```python
from build123d import *

# Parameters (mm, degrees)
ORIGINAL_TRUSS_PART_DEPTH = 30
SKETCH14_W                = 30
SKETCH14_H                = 30
CENTER_SUPPORT_DEPTH      = 305.758522
RIGHT_SUPPORT_REACH       = 302
SKETCH15_W                = 80
SKETCH15_H                = 30


with BuildPart() as part:
    # Sketch2 → Original Truss Part (new body)
    with BuildSketch(Plane.XY):
        Polygon((0, 0), (-928.915298157, 0), (-928.915298157, 27.120739154), (71.084701843, 27.120739154), (71.084701843, -32.879260846), (-8.915298157, -32.879260846), (-928.915298157, -330), (-928.915298157, -300), align=None)
    original_truss_part = extrude(amount=-ORIGINAL_TRUSS_PART_DEPTH)

    # OG Part Mirror: Original Truss Part across plane
    add(original_truss_part.mirror(Plane.ZX.offset(-152.879260846)))

    # Sketch14 → Center Support (add)
    with BuildSketch(Plane(origin=(0, -305.758521692, 0), x_dir=(1, 0, 0), z_dir=(0, 1, 0))):
        with Locations((-426.927182328, 15)):
            Rectangle(SKETCH14_W, SKETCH14_H)
    extrude(amount=CENTER_SUPPORT_DEPTH)

    # Right Support: up to this plane
    right_support_end = Plane(origin=(-8.915298157, -32.879260846, -30), z_dir=(0.307327428, -0.951603831, 0))
    # Sketch15 → Right Support (add, up to the surface)
    with BuildSketch(Plane(origin=(0, -272.879260846, 0), x_dir=(1, 0, 0), z_dir=(0, 1, 0)), mode=Mode.PRIVATE) as right_support_sk1:
        with Locations((31.084701843, 15)):
            Rectangle(SKETCH15_W, SKETCH15_H)
    right_support_tool1 = split(extrude(right_support_sk1.sketch, amount=RIGHT_SUPPORT_REACH, mode=Mode.PRIVATE), bisect_by=right_support_end, keep=Keep.BOTH, mode=Mode.PRIVATE)
    add(right_support_tool1.solids().sort_by_distance((31.084702, -272.879261, -15))[0])


solid = part.part
```
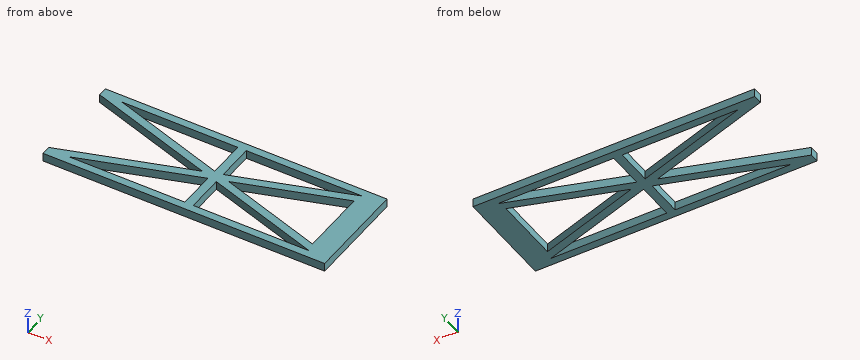
CAD build for the part. Positions are in the model's coordinates, mm. Give positions to 0.01 mm unless a question says otherwise; leave off trailing zeros. Order: outer loops, then holes, each group sorted by start corner. A loop starts at its lowest first (then second) coordinate and runs counter-clockwise, first axis right, second up.
(1) Saw through at C-C, the plane x = -559.5. Give the cut face in (y, z).
(2) Saw through at B-B, the plane y = -189. Give the cut face in (x, z), then the cut area to 3 significant figures.
(3) Saw through at A-A, the plane z = -10. Give the cut face in (x, y), then the cut area to 3 significant figures.
(4) Flat gauge pin, fed straight in: pin 1 (1 mm diameter, centred on x = -161, y = -58, fed in from +Z). Where does the tip first touch, or does it go through?
(5) Drill centre lines: L1, parallel to Y at x = -661, z = -7; L2, parallel to Y at x = -631, z = -17; L3, parallel to Y at x = -388, z = -9.75. Where is each one in solid material? Low to high.
Results found:
1. outline: (-332.88, -30) - (-305.76, -30) - (-305.76, 0) - (-332.88, 0) - close; (-210.69, -30) - (-180.69, -30) - (-180.69, 0) - (-210.69, 0) - close; (-125.06, -30) - (-95.06, -30) - (-95.06, 0) - (-125.06, 0) - close; (0, -30) - (27.12, -30) - (27.12, 0) - (0, 0) - close
2. outline: (-585.22, -30) - (-492.33, -30) - (-492.33, 0) - (-585.22, 0) - close; (-441.93, -30) - (-411.93, -30) - (-411.93, 0) - (-441.93, 0) - close; (-361.53, -30) - (-268.64, -30) - (-268.64, 0) - (-361.53, 0) - close; (-8.92, -30) - (71.08, -30) - (71.08, 0) - (-8.92, 0) - close
2. area: 8,870 mm2
3. outline: (-928.92, -332.88) - (71.08, -332.88) - (71.08, 27.12) - (-928.92, 27.12) - (-928.92, -5.76) - (-473.37, -152.88) - (-928.92, -300) - close; hole (-853.85, -305.76) - (-441.93, -305.76) - (-441.93, -172.72) - close; hole (-853.85, 0) - (-441.93, -133.03) - (-441.93, 0) - close; hole (-411.93, -305.76) - (0, -305.76) - (-411.93, -172.72) - close; hole (-411.93, -133.03) - (0, 0) - (-411.93, 0) - close; hole (-380.48, -152.88) - (-8.92, -272.88) - (-8.92, -32.88) - close
3. area: 139,000 mm2
4. pin 1: stops at z = 0
5. L1: y = -332.88 to -305.76, -243.47 to -213.47, -92.28 to -62.28, 0 to 27.12
5. L2: y = -332.88 to -305.76, -233.79 to -203.79, -101.97 to -71.97, 0 to 27.12
5. L3: y = -332.88 to -305.76, -180.45 to -125.31, 0 to 27.12
